from build123d import *

# Parameters (mm, degrees)
F0_W      = 50
F0_H      = 12.5
F1_DEPTH  = 8
F2_DEPTH  = 75
F4_DEPTH  = 8
F7_DEPTH  = 3
F8_DEPTH  = 1
F11_DEPTH = 3
F14_DEPTH = 3
F15_DEPTH = 8
F16_DEPTH = 25
F17_DEPTH = 8
F18_DEPTH = 8
F19_DEPTH = 8


# Not quite as in the source:
# - a feature names something its author has since deleted; it is built from what else it names


with BuildPart() as f1:
    # F0 (on Top) → F1 (new body)
    with BuildSketch(Plane.XY):
        Polygon((-42.0179491924, 72.7772228311), (-60.5095952989, 40.7487522591), (-57.9695070384, 39.3207329262), (-55.5194165334, 43.6791064608), (-50.2642610162, 40.7248836223), (-52.7144317239, 36.366367418), (-57.615009792, 27.6494680496), (-60.0654171506, 23.2910848888), (-65.3204122546, 26.2455930623), (-62.870004896, 30.6039762231), (-65.5097997054, 32.0881441788), (-84.0358983849, 0), (-42.0179491924, -72.7772228311), (42.0179491924, -72.7772228311), (84.0358983849, 0), (65.5442522784, 32.028470572), (63.0375071287, 30.542699277), (65.5869240764, 26.2416718908), (60.4009142911, 23.1676851313), (60.2621924773, 23.4017175915), (60.0654171506, 23.2910848888), (57.615009792, 27.6494680496), (55.164720758, 32.0079177338), (52.8483970279, 36.1280767392), (52.7526466281, 36.0713280944), (50.2033797707, 40.372634697), (50.3975781651, 40.4877307774), (50.2642610162, 40.7248836223), (55.5194165334, 43.6791064608), (57.9695070384, 39.3207329262), (60.5095952989, 40.7487522591), (42.0179491924, 72.7772228311), align=None)
        with Locations((0, 54.5829171234)):
            Rectangle(F0_W, F0_H, mode=Mode.SUBTRACT)
    extrude(amount=F1_DEPTH)

    # F0 (on Top) → F2 (join)
    with BuildSketch(Plane.XY):
        Polygon((-84.0358983849, 0), (-87.5, 0), (-43.75, -75.7772228311), (-4.799692811, -75.7772228311), (4.9533583678, -75.7772228311), (43.75, -75.7772228311), (87.5, 0), (84.0358983849, 0), (42.0179491924, -72.7772228311), (-42.0179491924, -72.7772228311), align=None)
    extrude(amount=F2_DEPTH)

    # F0 (on Top) → F4 (join)
    with BuildSketch(Plane.XY):
        Polygon((43.75, 75.7772228311), (-43.75, 75.7772228311), (-63.1248363216, 42.2190219338), (-60.5095952989, 40.7487522591), (-42.0179491924, 72.7772228311), (42.0179491924, 72.7772228311), (60.5095952989, 40.7487522591), (63.1248363216, 42.2190219338), align=None)
    extrude(amount=F4_DEPTH)

    # F6 (on face) → F7 (join)
    with BuildSketch(Plane(origin=(0, -50.1312366318, 89.3836679776), x_dir=(1, 0, 0), z_dir=(0, 0.4891706574, -0.872188092))):
        Polygon((43.75, 29.4041920927), (0, 29.4041920927), (-43.75, 29.4041920927), (-42.01795, -57.4775522498), (42.01795, -57.4775522498), align=None)
    extrude(amount=F7_DEPTH)

    # F3 (on Front) → F8 (join)
    with BuildSketch(Plane.XZ):
        Polygon((-42.01795, 114.5), (0, 114.5), (42.01795, 114.5), (84.0359, 75), (87.5, 75), (42.01795, 117.5), (0, 117.5), (-42.01795, 117.5), (-87.5, 75), (-84.0359, 75), align=None)
    extrude(amount=F8_DEPTH)

    # F10 (on face) → F11 (join)
    with BuildSketch(Plane(origin=(-67.6846727043, -39.0777640058, 72.4338274863), x_dir=(0.7723629594, -0.3015876344, 0.5590173143), z_dir=(-0.6351814378, -0.3667221741, 0.6797495039))):
        Polygon((33.2314262259, 55.789645187), (-25.6554603702, 35.6104118215), (30.9888924807, -31.0804218073), align=None)
    extrude(amount=-F11_DEPTH)

    # F13 (on face) → F14 (join)
    with BuildSketch(Plane(origin=(67.6756688636, -39.5950852503, 72.4241918832), x_dir=(0.7733047167, 0.3041472681, -0.556322078), z_dir=(-0.6340345536, 0.3709553614, -0.6785221475))):
        Polygon((-30.939509805, 30.5117392321), (-32.8751652468, -56.3649154418), (25.9400068576, -35.9776056011), align=None)
    extrude(amount=F14_DEPTH)

    # F0 (on Top) → F15 (join)
    with BuildSketch(Plane.XY):
        with Locations((0, 54.5829171234)):
            Rectangle(F0_W, F0_H)
    extrude(amount=F15_DEPTH)

    # F0 (on Top) → F16 (cut)
    with BuildSketch(Plane.XY):
        Polygon((-57.9695070384, 39.3207329262), (-60.5095952989, 40.7487522591), (-65.5097997054, 32.0881441788), (-62.870004896, 30.6039762231), (-57.615009792, 27.6494680496), (-52.7144317239, 36.366367418), align=None)
    extrude(amount=-F16_DEPTH, mode=Mode.SUBTRACT)

    # F0 (on Top) → F17 (join)
    with BuildSketch(Plane.XY):
        Polygon((-65.5097997054, 32.0881441788), (-68.125, 33.5584843966), (-87.5, 0), (-84.0358983849, 0), align=None)
        Polygon((87.5, 0), (68.1251636784, 33.5582008974), (65.5442522784, 32.028470572), (84.0358983849, 0), align=None)
    extrude(amount=F17_DEPTH)

    # F0 (on Top) → F18 (join)
    with BuildSketch(Plane.XY):
        Polygon((4.9533583678, -75.7772228311), (-4.799692811, -75.7772228311), (-4.8760764436, -82.0772228311), (-4.9366983742, -87.0772228311), (-4.8147415831, -87.0772228311), (4.8147415831, -87.0772228311), (4.8760764436, -82.0772228311), align=None)
        Polygon((9.3760764436, -82.0772228311), (4.8760764436, -82.0772228311), (4.8147415831, -87.0772228311), (9.3147415831, -87.0772228311), align=None)
    extrude(amount=F18_DEPTH)

    # F0 (on Top) → F19 (join)
    with BuildSketch(Plane.XY):
        Polygon((-4.9366983742, -87.0772228311), (-4.8760764436, -82.0772228311), (-9.3760764436, -82.0772228311), (-9.3147415831, -87.0772228311), align=None)
    extrude(amount=F19_DEPTH)


solid = f1.part
CAD build for the part. Positions are in the model's coordinates, mm. A direction names the side the tool comes from. Give positions to 0.01 mm unless a question says otherwise; leave off trailing zeros. Write each loop counter-clockwise with the first axis right and the second up, starting at its lowest first coordinate (ties: lowest second). Pieces come first, ordered by that corner, then holes. Notation, with made-up numbers: M 83,56.5 L 112,56.5 A16 ccw 112,87.5 Z; hole C -2,-30.75 d8. An arc over 180 degrees is marked long. Put each result on its own line as item: value. Start each with the question number.
(1) Probe L1, parallel to Y at x = 2, z = 42; L2, parallel to X at y = -30, z = 18; L3, parallel to Z at x = 36, y = -2.5. List the from-to ranges inside material, lowest first.
(2) Which spindle directions (+Z, -Z, +X, -X, +Y, -Y) get a long thin tool onto all of the face, cutting with end or side? Do faces 4 (the face through (-7, -82.077, 4)), 5 (the face through (0, -83, 8)), 6 (the face through (-56.76, 41.47, 3.94)), 7 (the face through (-53.7, -22, 90.3)), 8 (the face through (53.573, 58.763, 3.944)). Say none if no direction does.
(3) Mould opens along Y. For faces 1 (the face through (-0.586, -36.175, 93.772)), 2 (the face through (-65.93, -37.36, 36.98)), 3 (the face through (-52.929, 42.223, 3.944)) say: +Y half, -Y half, draft (parallel to the pull), parting line (faces both ways), or undercut.
(4) Band-saw the part on A-A, the plane x = -20. Write the cut outline in (y, z).
(5) Band-saw the part on D-D, the plane y = -61. Write the cut outline in (x, z).
(6) Band-saw the part on B-B, the plane z = 36. Write the cut outline in (x, y).
(7) Flat gauge pins, fed straight in: pin 1 Ø4 at (x, z) = (-86.5, 49.5) entering from +Y; pin 2 Ø2 at (y, z) = (-11, 42) entering from +X; pin 3 Ø3 at (y, z) = (-37, 15.5) entering from +X; pin 4 Ø1 at (x, y) = (-63, 27) entering from +Z. Where does each tip first touch, or does it go through?
(8) Band-saw the part on C-C, the plane y = -28. Write the cut outline in (x, z).
Response values:
1. L1: y = -75.78 to -72.78
1. L2: x = -70.18 to -66.72, 66.72 to 70.18
1. L3: z = 0 to 8, 112.66 to 116.1
2. face 4: +Z, -Z, -X
2. face 5: +Z, +X, -X, -Y
2. face 6: +Z, -Z
2. face 7: +Y
2. face 8: +Z, -Z, +X, +Y
3. face 1: +Y half
3. face 2: -Y half
3. face 3: undercut
4. outline: M -75.78,0 L 75.78,0 L 75.78,8 L -72.78,8 L -72.78,73.24 L 1.47,114.88 L 0,117.5 L -1,117.5 L -1,116.94 L -75.78,75 Z
5. outline: M -52.28,0 L 52.28,0 L 52.28,75 L 52.34,75.05 L 43.46,83.35 L 43.41,83.29 L -43.41,83.29 L -52.28,75 Z; hole M -48.82,8 L 48.82,8 L 48.82,73.92 L 42.48,79.85 L -42.37,79.85 L -48.82,73.82 Z
6. outline: M -87.5,0 L -43.75,-75.78 L 43.75,-75.78 L 87.5,0 L 84.04,0 L 42.02,-72.78 L -42.02,-72.78 L -84.04,0 Z
7. pin 1: stops at y = 0
7. pin 2: stops at x = 81.73
7. pin 3: stops at x = 67
7. pin 4: passes through
8. outline: M -71.33,0 L 71.33,0 L 71.33,75 L 71.53,75.16 L 42.8,102 L 42.66,101.8 L -42.66,101.8 L -71.33,75 Z; hole M -67.87,8 L 67.87,8 L 67.87,74.16 L 41.98,98.36 L -41.62,98.36 L -67.87,73.82 Z
